Geometry check sheet. Reference: the model listing, model coordinates, mm. A direction names the side the tool comes from. Round coordinates to 2 decimals unless told otherwise and drop trailing zeros. Order: outer loops, then holes, each group sorted by start corner. A loop starts at its lowest first (then second) coordinate and runs counter-clockwise, first axis right, second up. Notation, with made-up numbers: (-31, 35.25) - (22, 35.25) arc R13 ccw to (22, 41.25) - close; hole circle Ø10 at (23, 19). An arc over 180 degrees is marked (long way). Use a Markdown table: item, result. Add a question column.
(1) Section check A-A on y = -3. Record the boundary of the cut face in (x, z).
(2) Access from +Z, -Z, +X, -X, +Y, -Y to the whole of each face (thin tool, end or side, straight path). Record for faces 1 (the face through (-6.834, -0.208, -1.517)), 2 (the face through (0.1, 24.15, 4.4)).
(3) Gauge pin test, flat ends, axial feed: P1, Ø6, axis at x = -4, y = 1.5, coming from the +Z side; P2, Ø8, axis at y = 9.5, z = 5.5, coming from the +X side; P3, Ø1.5, axis at x = -4, y = 18.5, coming from the +Z side. Record the tip position at first contact, or that the pin passes through.
(4) Thickness scan on line 1 along Y through (x, z) = (2.25, 5.75); line 2 along Y through (x, z) = (-2, -1.75); line 3 along Z through (x, y) = (-0.75, 4). Record the ranges inside material, lowest first. Write a range as [from, to].
```python
from build123d import *

# Parameters (mm, degrees)
BOSS_EXTRUDE1_DEPTH      = 24.15
BOSS_EXTRUDE1_DEPTH_BACK = 24.15
SKETCH1_R                = 7
FILLET1_R                = 0.5
CHAMFER1_SIZE            = 0.25
SKETCH2_R                = 4.25
BOSS_EXTRUDE2_DEPTH      = 0.1
FILLET2_R                = 0.1
SKETCH3_R                = 2.5
BOSS_EXTRUDE3_DEPTH      = 1
FILLET3_R                = 0.2
FILLET4_R                = 0.2


with BuildPart() as part:
    # Sketch1 → Boss-Extrude1 (new, two sides: drawn at the far end of the back side and taken through both)
    with BuildSketch(Plane(origin=(0, 0, 0), x_dir=(1, 0, 0), z_dir=(0, 1, 0)).offset(-BOSS_EXTRUDE1_DEPTH_BACK)):
        with Locations(Location((0, 0, 0), (0, 0, 270))):
            Circle(SKETCH1_R)
    extrude(amount=BOSS_EXTRUDE1_DEPTH + BOSS_EXTRUDE1_DEPTH_BACK)

    # Fillet1
    fillet1_edges = [part.edges().sort_by_distance(p)[0] for p in [
        (0, -24.15, -7),
    ]]
    fillet(fillet1_edges, radius=FILLET1_R)

    # Chamfer1
    chamfer1_edges = [part.edges().sort_by_distance(p)[0] for p in [
        (0, 24.15, -7),
    ]]
    chamfer(chamfer1_edges, length=CHAMFER1_SIZE)

    # Sketch2 → Boss-Extrude2 (add)
    with BuildSketch(Plane(origin=(0, 24.15, 0), x_dir=(1, 0, 0), z_dir=(0, 1, 0))):
        with Locations(Location((0, 0, 0), (0, 0, 270))):
            Circle(SKETCH2_R)
    extrude(amount=BOSS_EXTRUDE2_DEPTH)

    # Fillet2
    fillet2_edges = [part.edges().sort_by_distance(p)[0] for p in [
        (0, 24.25, -4.25),
    ]]
    fillet(fillet2_edges, radius=FILLET2_R - 0.0001)  # a hair under: the kernel refuses the full size

    # Sketch3 → Boss-Extrude3 (add)
    with BuildSketch(Plane(origin=(0, 24.25, 0), x_dir=(1, 0, 0), z_dir=(0, 1, 0))):
        with Locations(Location((0, 0, 0), (0, 0, 270))):
            Circle(SKETCH3_R)
    extrude(amount=BOSS_EXTRUDE3_DEPTH)

    # Fillet3
    fillet3_edges = [part.edges().sort_by_distance(p)[0] for p in [
        (0, 24.25, -2.5),
    ]]
    fillet(fillet3_edges, radius=FILLET3_R)

    # Fillet4
    fillet4_edges = [part.edges().sort_by_distance(p)[0] for p in [
        (0, 25.25, -2.5),
    ]]
    fillet(fillet4_edges, radius=FILLET4_R)


solid = part.part
```
Check sheet entries:
| question | item | result |
|---|---|---|
| 1 | outline | circle Ø14 at (0, 0) |
| 2 | face 1 | +Y, -Y |
| 2 | face 2 | +Y |
| 3 | P1 | stops at z = 6.93 |
| 3 | P2 | stops at x = 6.84 |
| 3 | P3 | stops at z = 6.2 |
| 4 | line 1 | y = [-24.15, 24.15] |
| 4 | line 2 | y = [-24.15, 24.25] |
| 4 | line 3 | z = [-6.96, 6.96] |
